```python
from build123d import *

# Parameters (mm, degrees)
SKETCH2_W               = 44
SKETCH2_H               = 47
BOSS_EXTRUDE1_DEPTH     = 3.5
SKETCH3_W               = 44
SKETCH3_H               = 22.5
BOSS_EXTRUDE2_DEPTH     = 10.5
SKETCH4_W               = 23
SKETCH4_H               = 15.5
BOSS_EXTRUDE3_DEPTH     = 25.5
SKETCH5_W               = 6.5
SKETCH5_H               = 8
SKETCH5_W_2             = 6
CUT_EXTRUDE1_DEPTH      = 10.5
SKETCH6_R               = 1.5
CUT_EXTRUDE3_DEPTH      = 30
CUT_EXTRUDE3_DEPTH_BACK = 1


with BuildPart() as part:
    # Sketch2 → Boss-Extrude1 (new body)
    with BuildSketch(Plane(origin=(0, 0, 0), x_dir=(1, 0, 0), z_dir=(0, 1, 0))):
        with Locations((22, 23.5)):
            Rectangle(SKETCH2_W, SKETCH2_H)
    extrude(amount=BOSS_EXTRUDE1_DEPTH)

    # Sketch3 → Boss-Extrude2 (add)
    with BuildSketch(Plane(origin=(0, 3.5, 0), x_dir=(1, 0, 0), z_dir=(0, 1, 0))):
        with Locations((22, 15.75)):
            Rectangle(SKETCH3_W, SKETCH3_H)
    extrude(amount=BOSS_EXTRUDE2_DEPTH)

    # Sketch4 → Boss-Extrude3 (add)
    with BuildSketch(Plane(origin=(0, 3.5, 0), x_dir=(1, 0, 0), z_dir=(0, 1, 0))):
        with Locations((21.5, 39.25)):
            Rectangle(SKETCH4_W, SKETCH4_H)
    extrude(amount=BOSS_EXTRUDE3_DEPTH)

    # Sketch5 → Cut-Extrude1 (cut)
    with BuildSketch(Plane(origin=(0, 14, 0), x_dir=(1, 0, 0), z_dir=(0, 1, 0))):
        with Locations((3.25, 8.5)):
            Rectangle(SKETCH5_W, SKETCH5_H)
        with Locations((41, 8.5)):
            Rectangle(SKETCH5_W_2, SKETCH5_H)
    extrude(amount=-CUT_EXTRUDE1_DEPTH, mode=Mode.SUBTRACT)

    # Sketch6 → Cut-Extrude3 (cut, two sides)
    with BuildSketch(Plane(origin=(0, 0, 0), x_dir=(1, 0, 0), z_dir=(0, 1, 0))) as cut_extrude3_sk:
        with Locations((3.1, 43.9)):
            Circle(SKETCH6_R)
        with Locations((40.9, 43.9)):
            Circle(SKETCH6_R)
        with Locations((40.9, 4.6)):
            Circle(SKETCH6_R)
        with Locations((3.1, 4.6)):
            Circle(SKETCH6_R)
    extrude(amount=CUT_EXTRUDE3_DEPTH, mode=Mode.SUBTRACT)
    extrude(cut_extrude3_sk.sketch, amount=-CUT_EXTRUDE3_DEPTH_BACK, mode=Mode.SUBTRACT)


solid = part.part
```
The listing builds one solid part. Answer for the finished solid, in the listing's coordinates (mm). A direction names the side the tool comes from. Coordinates: 2 decimals unless noted, no trailing zeros. Loops run counter-clockwise (first coordinate to the right, second up) from the corner with the lowest first, then second, coordinate; pieces in that order, holes last. Notation, with made-up numbers: (50, 16) - (84, 16) arc R12 ccw to (84, 34) - close; hole circle Ø4 at (21, -18). An arc over 180 degrees is marked (long way). Use a Markdown table: item, result. Add a question column.
1) The part is cut by section B-B, the plane z = -43.9. Give the vertices of the cut face in (x, y).
2) The part is cut by section C-C, the plane x = 3.1. Give the vertices of the cut face in (y, z).
3) Given pin 1 (12.5 mm diameter, centred on y = 22.5, z = -38.5, fed in from -X); pin 2 (8 mm diameter, centred on y = 10, z = -36.5, fed in from +X); pin 3 (1 mm diameter, centred on y = 6.5, z = -5.5, fed in from +X), each flat-ended and moving along its own axis, determine where each tip first touches the part or whether it passes through.
4) Find the intervals of material crossed by line 1 (Z direction, x = 3.1, y = 1.6); line 2 (X direction, y = 2.1, z = -4.6); line 3 (Z direction, x = 28, y = 12.25), in increasing order.
5) The part is cut by section D-D, the plane z = -38.5. Give the vertices of the cut face in (x, y).
6) The mould has two halves that part along Z. Classify faces 1 (the flat face through (22, 3.5, -4)), 2 (the flat face through (41, 9, -12.5)), 3 (the flat face through (22, 14, -47)), 4 (the flat face through (22, 3.5, -30)): released by +Z, released by -Z, zero draft, split by the parting line, or undercut.
7) The part is cut by section A-A, the plane y = 12. Give the vertices of the cut face in (x, z), and give its area (3 significant figures).
8) For faces 5 (the flat face through (21, 16, -31.5)), 6 (the flat face through (38, 9, -8)), 7 (the flat face through (10, 16, -39)), determine the directions among +Z, -Z, +X, -X, +Y, -Y from which every point of the face is accessible in a straight line to the end or side of a thin tool.
Here are the results:
| question | item | result |
|---|---|---|
| 1 | outline | (0, 0) - (1.6, 0) - (1.6, 3.5) - (0, 3.5) - close; (4.6, 0) - (39.4, 0) - (39.4, 3.5) - (33, 3.5) - (33, 29) - (10, 29) - (10, 3.5) - (4.6, 3.5) - close; (42.4, 0) - (44, 0) - (44, 3.5) - (42.4, 3.5) - close |
| 2 | outline | (0, -47) - (3.5, -47) - (3.5, -45.4) - (0, -45.4) - close; (0, -42.4) - (3.5, -42.4) - (3.5, -27) - (14, -27) - (14, -12.5) - (3.5, -12.5) - (3.5, -6.1) - (0, -6.1) - close; (0, -3.1) - (3.5, -3.1) - (3.5, 0) - (0, 0) - close |
| 3 | pin 1 | stops at x = 10 |
| 3 | pin 2 | stops at x = 33 |
| 3 | pin 3 | stops at x = 38 |
| 4 | line 1 | z = -47 to -45.4, -42.4 to -6.1, -3.1 to 0 |
| 4 | line 2 | x = 0 to 1.6, 4.6 to 39.4, 42.4 to 44 |
| 4 | line 3 | z = -47 to -31.5, -27 to -4.5 |
| 5 | outline | (0, 0) - (44, 0) - (44, 3.5) - (33, 3.5) - (33, 29) - (10, 29) - (10, 3.5) - (0, 3.5) - close |
| 6 | face 1 | zero draft |
| 6 | face 2 | released by +Z |
| 6 | face 3 | released by -Z |
| 6 | face 4 | undercut |
| 7 | outline | (0, -27) - (44, -27) - (44, -12.5) - (38, -12.5) - (38, -4.5) - (6.5, -4.5) - (6.5, -12.5) - (0, -12.5) - close; (10, -47) - (33, -47) - (33, -31.5) - (10, -31.5) - close |
| 7 | area | 1,250 mm^2 |
| 8 | face 5 | +X, -X, +Y |
| 8 | face 6 | +Z, +X, +Y |
| 8 | face 7 | -Z, -X, +Y |
